Autodesk Fusion 360 part; units mm, degrees
sketch "草图1" plane through (0, 0, 0) normal (0, 0, 1) x (1, 0, 0)
  line L0 (22.5, -15) -> (-22.5, -15)
  line L1 (-22.5, -15) -> (-22.5, 15)
  line L2 (-22.5, 15) -> (22.5, 15)
  line L3 (22.5, 15) -> (22.5, -15)
  line L4 (22.5, -15) -> (-22.5, 15) construction
  line L5 (-22.5, -15) -> (22.5, 15) construction
  dimension "d27" = 45
  dimension "d28" = 30
extrude "拉伸1" add sketch "草图1" along normal blind 6
sketch "草图2" plane through (0, 0, 0) normal (1, 0, 0) x (0, 1, 0)
sketch "草图3" plane through (0, 0, 0) normal (1, 0, 0) x (0, 1, 0)
  circle A0 centre (5, 6) radius 1.3
  dimension "d31" = 2.6
extrude "拉伸2" add sketch "草图3" along normal blind 12.5 and the other way blind 12.5
mirror "镜像1" about plane through (0, 0, 0) normal (0, 1, 0) of "拉伸2"
sketch "草图4" plane through (0, 0, 6) normal (0, 0, 1) x (-1, 0, 0)
  line L0 (12.5, 6.3) -> (12.5, 3.7)
  line L1 (12.5, 3.7) -> (-12.5, 3.7)
  line L2 (-12.5, 3.7) -> (-12.5, 6.3)
  line L3 (-12.5, 6.3) -> (12.5, 6.3)
  line L4 (12.5, -3.7) -> (12.5, -6.3)
  line L5 (12.5, -6.3) -> (-12.5, -6.3)
  line L6 (-12.5, -6.3) -> (-12.5, -3.7)
  line L7 (-12.5, -3.7) -> (12.5, -3.7)
  line L8 (-22.5, -15) -> (22.5, -15)
  line L9 (22.5, -15) -> (22.5, 15)
  line L10 (22.5, 15) -> (-22.5, 15)
  line L11 (-22.5, 15) -> (-22.5, -15)
fillet "圆角1" radius 2 4 edges at (22.5, 15, 3) (22.5, -15, 3) (-22.5, -15, 3) (-22.5, 15, 3)
sketch "草图5" plane through (0, 0, 6) normal (0, 0, 1) x (-1, 0, 0)
  line L0 (12.5, 6.3) -> (12.5, 3.7)
  line L1 (12.5, 3.7) -> (-12.5, 3.7)
  line L2 (-12.5, 3.7) -> (-12.5, 6.3)
  line L3 (-12.5, 6.3) -> (12.5, 6.3)
  line L4 (12.5, -3.7) -> (12.5, -6.3)
  line L5 (12.5, -6.3) -> (-12.5, -6.3)
  line L6 (-12.5, -6.3) -> (-12.5, -3.7)
  line L7 (-12.5, -3.7) -> (12.5, -3.7)
  arc A0 (20.5, -15) -> (22.5, -13) centre (20.5, -13) ccw
  line L8 (22.5, -13) -> (22.5, 13)
  arc A1 (22.5, 13) -> (20.5, 15) centre (20.5, 13) ccw
  line L9 (20.5, 15) -> (-20.5, 15)
  arc A2 (-20.5, 15) -> (-22.5, 13) centre (-20.5, 13) ccw
  line L10 (-22.5, 13) -> (-22.5, -13)
  arc A3 (-22.5, -13) -> (-20.5, -15) centre (-20.5, -13) ccw
  line L11 (-20.5, -15) -> (20.5, -15)
  circle A4 centre (-17, 10) radius 2.4
  dimension "d44" = 4.8
extrude "拉伸4" cut sketch "草图5" against normal blind 4 contours A4
sketch "草图6" plane through (0, 0, 6) normal (0, 0, 1) x (-1, 0, 0)
  circle A0 centre (-17, 10) radius 2.4
  line L0 (12.5, 6.3) -> (12.5, 3.7)
  line L1 (12.5, 3.7) -> (-12.5, 3.7)
  line L2 (-12.5, 3.7) -> (-12.5, 6.3)
  line L3 (-12.5, 6.3) -> (12.5, 6.3)
  line L4 (12.5, -3.7) -> (12.5, -6.3)
  line L5 (12.5, -6.3) -> (-12.5, -6.3)
  line L6 (-12.5, -6.3) -> (-12.5, -3.7)
  line L7 (-12.5, -3.7) -> (12.5, -3.7)
  arc A1 (20.5, -15) -> (22.5, -13) centre (20.5, -13) ccw
  line L8 (22.5, -13) -> (22.5, 13)
  arc A2 (22.5, 13) -> (20.5, 15) centre (20.5, 13) ccw
  line L9 (20.5, 15) -> (-20.5, 15)
  arc A3 (-20.5, 15) -> (-22.5, 13) centre (-20.5, 13) ccw
  line L10 (-22.5, 13) -> (-22.5, -13)
  arc A4 (-22.5, -13) -> (-20.5, -15) centre (-20.5, -13) ccw
  line L11 (-20.5, -15) -> (20.5, -15)
  circle A5 centre (17, -10) radius 2.4
  dimension "d47" = 4.8
extrude "拉伸5" cut sketch "草图6" against normal blind 4 contours A5
equation "Catheter_Diameter = Flexible spring catheter outer diameter"
equation "Catheter_Assembly_Clearance = Initial diametral assembly clearance between catheter and Ecoflex liner"
equation "Clamp_Groove_Diameter = Hard clamp circular groove diameter"
equation "Pad_Outer_Diameter = Ecoflex liner outer diameter driven by clamp groove"
equation "Pad_Outer_Radius = Ecoflex liner outer radius"
equation "Pad_Inner_Diameter = Ecoflex liner inner diameter"
equation "Pad_Inner_Radius = Ecoflex liner inner radius"
equation "Pad_Radial_Thickness = Nominal radial thickness of Ecoflex liner"
equation "Pad_Length = Effective Ecoflex liner length"
equation "Mold_Length = Overall mold length along X"
equation "Mold_Width = Overall mold width along Y"
equation "Bottom_Mold_Thickness = Bottom mold plate thickness"
equation "Top_Mold_Thickness = Top mold plate thickness"
equation "Top_Mold_Base_Z = Assembly Z height of top mold bottom parting face"
equation "Pad_Cavity_Offset_Y = Centerline offset of the two cavities from mold center"
equation "Alignment_Pin_Diameter = Printed alignment pin diameter on bottom mold"
equation "Alignment_Pin_Height = Alignment pin height"
equation "Alignment_Hole_Diameter = Alignment blind-hole diameter on top mold"
equation "Alignment_Hole_Depth = Alignment blind-hole depth"
equation "Alignment_Pin_Offset_X = Absolute X coordinate magnitude of alignment pins"
equation "Alignment_Pin_Offset_Y = Absolute Y coordinate magnitude of alignment pins"
equation "Overflow_Channel_Width = Optional V1 overflow-channel width; retained but not used in recommended V1"
equation "Overflow_Channel_Depth = Optional V1 overflow-channel depth; retained but not used in recommended V1"
equation "Overflow_Well_Diameter = Optional overflow-well diameter; retained but not used in recommended V1"
equation "Overflow_Well_Depth = Optional overflow-well depth; retained but not used in recommended V1"
equation "Mold_Outer_Fillet = External handling-edge fillet radius"
equation "d27 = Mold_Length"
equation "d28 = Mold_Width"
equation "d29 = Top_Mold_Thickness"
equation "d31 = Pad_Inner_Diameter"
equation "d32 = Pad_Length / 2"
equation "d34 = Pad_Length / 2"
equation "d43 = Mold_Outer_Fillet"
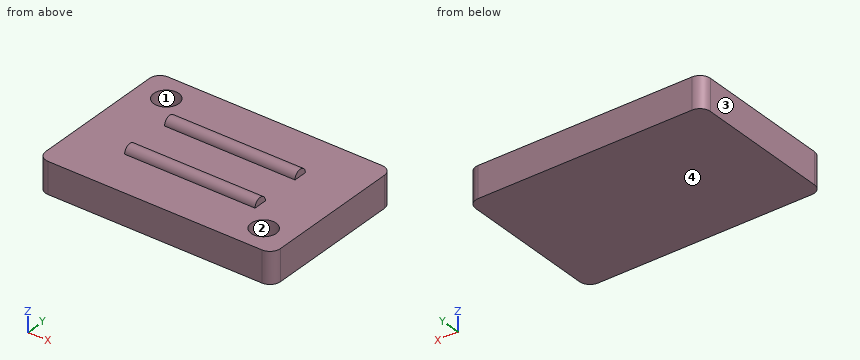
Build history of the part. All positions in model axes, mm. Face numbers are marked on the shaded views. Give positions to 0.01 mm unless a question says otherwise; leave off trailing zeros. Order: outer loops, then holes, each group sorted by start corner. A loop starts at its lowest first (then second) coordinate and runs counter-clockwise, first axis right, second up. Notation, with made-up numbers: M 10.5,-10 L 52.5,-10 A13 ccw 52.5,1 Z; hole C 61,-3.75 d4. An arc over 180 degrees is marked long. Return JSON: item names as keys, results as strings.
Q1. Band-saw the part on A-A (z = 5.5). Give the cut face in (x, y), then the cut area to 3 significant figures.
Answer list:
{"outline": "M -22.5,-13 A2 ccw -20.5,-15 L 20.5,-15 A2 ccw 22.5,-13 L 22.5,13 A2 ccw 20.5,15 L -20.5,15 A2 ccw -22.5,13 Z; hole C -17,10 d4.8; hole C 17,-10 d4.8", "area": "1,310 mm^2"}
Q2. Band-saw the part on C-C (x = -17). Give the cut face in (y, z), then the cut area to 3 significant figures.
Answer list:
{"outline": "M -15,0 L 15,0 L 15,6 L 12.4,6 L 12.4,2 L 7.6,2 L 7.6,6 L -15,6 Z", "area": "161 mm^2"}
Q3. Flat gauge pins, fed straight in: pin 1 (4 mm diameter, centred on x = -18, y = 10.5, fed in from +Z); pin 2 (3 mm diameter, centred on x = 17, y = -10, fed in from +Z); pin 3 (0.6 mm diameter, centred on y = -4.5, z = 6.5, fed in from +X). Where does each tip first touch, or does it go through?
Answer list:
{"pin 1": "stops at z = 6", "pin 2": "stops at z = 2", "pin 3": "stops at x = 12.5"}
Q4. Two-plate mould, pull along X, no slides. Class the marked faces 1, 2, 3 and 4: pulls with the +X half, pulls with the -X half, needs draft (parallel to the pull), parting line crosses it, or undercut.
Answer list:
{"face 1": "undercut", "face 2": "undercut", "face 3": "pulls with the -X half", "face 4": "needs draft"}
Q5. Band-saw the part on D-D (y = 1.75). Give the cut face in (x, z), then the cut area to 3 significant figures.
Answer list:
{"outline": "M -22.5,0 L 22.5,0 L 22.5,6 L -22.5,6 Z", "area": "270 mm^2"}
Q6. Wall check: probe 1 along X at (y, z) = (10, 4); probe 2 along Y at (x, z) = (17, 3.05); probe 3 along X at (y, z) = (-10, 4). Give the ranges that are in metal, low to high. Write a range as from..to.
Answer list:
{"probe 1": "x = -22.5..-19.4, -14.6..22.5", "probe 2": "y = -15..-12.4, -7.6..15", "probe 3": "x = -22.5..14.6, 19.4..22.5"}
Q7. Band-saw the part on B-B (y = 5). Give the cut face in (x, z).
Answer list:
{"outline": "M -22.5,0 L 22.5,0 L 22.5,6 L 12.5,6 L 12.5,7.3 L -12.5,7.3 L -12.5,6 L -22.5,6 Z"}
